Verification items for this drawing (mm, ordinates from the low corner). Coordinates: 2 decimals unless noted, no trailing zeros. Write each loop counter-clockwise with the first axis right and the second up, starting at its lowest first coordinate (ties: lowest second). Pieces come first, ordered by that corner, then holes. Notation, with made-up numbers: M -23.75,42.5 L 6.25,42.5 A25 cw 6.25,62.5 Z; hole C 40,74 d8. An arc over 180 degrees is marked long. Put each result on its own line as item: value. Start each with the question number.
1) Scan lines: line 1 along X through (y, z) = (1.5, 52.5); line 2 along Z through (x, y) = (28.5, 1.85) (1 decimal); line 3 along Z through (x, y) = (28.75, 2.2) (1 decimal). Record each from-to range of solid material in increasing order.
2) Cross-section at A-A on z = 32. Record the cut outline in (x, y).
3) Gauge pin test, flat ends, axial feed: pin 1 (4 mm diameter, centred on x = 100, z = 52.5, fed in from +Y); pin 2 (3 mm diameter, centred on x = 93.64, z = 28.75, fed in from +Y); pin 3 (1.5 mm diameter, centred on y = 3, z = 89.5, fed in from +X); pin 4 (12 mm diameter, centred on x = 65, z = 85, fed in from +Y). Record the tip position at first contact, or that the pin passes through.
4) Cross-section at D-D on x = 28.75. Record the cut outline in (y, z).
5) Cross-section at C-C on y = 2.75. Count the separate pieces of the cut face and the enclosed holes in it, plus the area to 4 significant figures.
6) Cross-section at B-B on x = 60. Record the cut outline in (y, z), plus the area to 3 significant figures.
7) Mould release check, pull along X, two halves, no side actions. Record for the marked faces 1 and 2: released by +X, released by -X, zero draft, split by the parting line, or undercut.
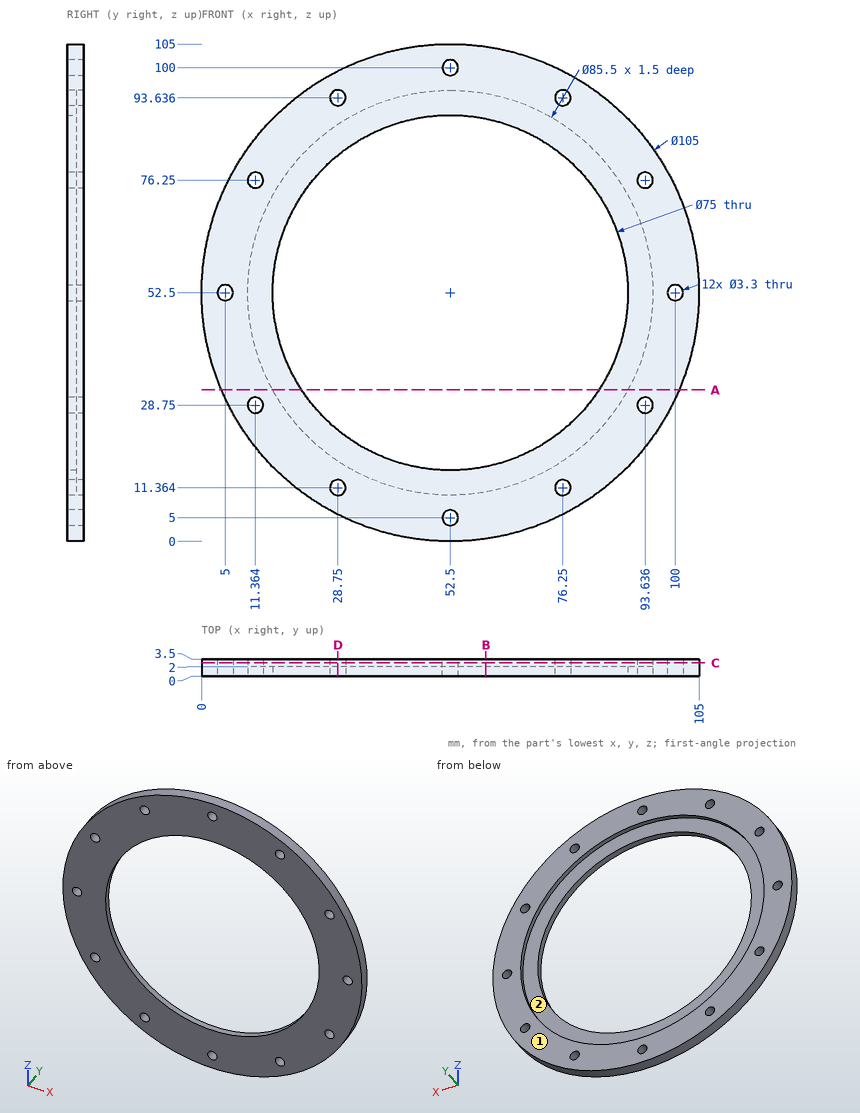
Answer key:
1. line 1: x = 0 to 3.35, 6.65 to 15, 90 to 98.35, 101.65 to 105
1. line 2: z = 5.8 to 9.7, 13 to 23.7, 81.3 to 92, 95.3 to 99.2
1. line 3: z = 5.7 to 9.7, 13 to 17, 88 to 92, 95.3 to 99.3
2. outline: M 4.17,0 L 21.1,0 L 21.1,2 L 14.99,2 L 14.99,3.5 L 4.17,3.5 Z; M 83.9,0 L 100.83,0 L 100.83,3.5 L 90.01,3.5 L 90.01,2 L 83.9,2 Z
3. pin 1: stops at y = 3.5
3. pin 2: passes through
3. pin 3: stops at x = 90.48
3. pin 4: stops at y = 2
4. outline: M 0,5.68 L 3.5,5.68 L 3.5,9.71 L 0,9.71 Z; M 0,13.01 L 3.5,13.01 L 3.5,16.95 L 2,16.95 L 2,23.48 L 0,23.48 Z; M 0,81.52 L 2,81.52 L 2,88.05 L 3.5,88.05 L 3.5,91.99 L 0,91.99 Z; M 0,95.29 L 3.5,95.29 L 3.5,99.32 L 0,99.32 Z
5. separate pieces: 1
5. enclosed holes: 13
5. area: 2,815 mm²
6. outline: M 0,0.54 L 3.5,0.54 L 3.5,10.41 L 2,10.41 L 2,15.76 L 0,15.76 Z; M 0,89.24 L 2,89.24 L 2,94.59 L 3.5,94.59 L 3.5,104.46 L 0,104.46 Z
6. area: 90.5 mm²
7. face 1: zero draft
7. face 2: undercut
